Geometry: final body of the model. Coordinates: model frame, mm. A direction names the side the tool comes from. Round coordinates to 2 decimals unless told otherwise and drop trailing zeros. Loops run counter-clockwise (first coordinate to the right, second up) from the corner with the lowest first, then second, coordinate; pieces in that order, holes last. Notation, with made-up numbers: (67.25, 4) - (126.25, 4) arc R24 ccw to (126.25, 40) - close; hole circle Ø5 at (-21.75, 76.5). An arc over 180 degrees is marked (long way). Answer as CSV lines item,"result".
from build123d import *

# Parameters (mm, degrees)
SKETCH1_W           = 76.2
SKETCH1_H           = 50.8
BOSS_EXTRUDE2_DEPTH = 1016
SKETCH2_R           = 25.4
CUT_EXTRUDE1_DEPTH  = 1016
FILLET1_R           = 25.4
SKETCH3_R           = 12.7
CUT_EXTRUDE2_DEPTH  = 254
SKETCH4_W           = 38.1
SKETCH4_H           = 50.8
CUT_EXTRUDE3_DEPTH  = 254
SKETCH5_W           = 38.1
SKETCH5_H           = 25.4
CUT_EXTRUDE4_DEPTH  = 254
FILLET2_R           = 25.4


with BuildPart() as part:
    # Sketch1 → Boss-Extrude2 (new body)
    with BuildSketch(Plane(origin=(0, 0, 0), x_dir=(1, 0, 0), z_dir=(0, 1, 0))):
        with Locations((38.1, -25.4)):
            Rectangle(SKETCH1_W, SKETCH1_H)
    extrude(amount=BOSS_EXTRUDE2_DEPTH)

    # Sketch2 → Cut-Extrude1 (cut)
    with BuildSketch(Plane.XY.offset(50.8)):
        with Locations((38.1, 965.2)):
            Circle(SKETCH2_R)
    extrude(amount=-CUT_EXTRUDE1_DEPTH, mode=Mode.SUBTRACT)

    # Fillet1
    fillet1_edges = [part.edges().sort_by_distance(p)[0] for p in [
        (76.2, 1016, 25.4),
        (0, 1016, 25.4),
    ]]
    fillet(fillet1_edges, radius=FILLET1_R)

    # Sketch3 → Cut-Extrude2 (cut)
    with BuildSketch(Plane.XY.offset(50.8)):
        with Locations((38.1, 25.4)):
            Circle(SKETCH3_R)
    extrude(amount=-CUT_EXTRUDE2_DEPTH, mode=Mode.SUBTRACT)

    # Sketch4 → Cut-Extrude3 (cut)
    with BuildSketch(Plane.ZY):
        with Locations((25.4, 25.4)):
            Rectangle(SKETCH4_W, SKETCH4_H)
    extrude(amount=-CUT_EXTRUDE3_DEPTH, mode=Mode.SUBTRACT)

    # Sketch5 → Cut-Extrude4 (cut)
    with BuildSketch(Plane.ZY):
        with Locations((25.4, 63.5)):
            Rectangle(SKETCH5_W, SKETCH5_H)
    extrude(amount=-CUT_EXTRUDE4_DEPTH, mode=Mode.SUBTRACT)

    # Fillet2
    fillet2_edges = [part.edges().sort_by_distance(p)[0] for p in [
        (0, 0, 47.625),
        (76.2, 0, 3.175),
        (76.2, 0, 47.625),
        (0, 0, 3.175),
    ]]
    fillet(fillet2_edges, radius=FILLET2_R)


solid = part.part
(1) Section C-C (x = 38.1). Output: boundary loops of the cut face in (y, z).
Findings below:
outline,"(0, 0) - (12.7, 0) - (12.7, 6.35) - (0, 6.35) - close; (0, 44.45) - (12.7, 44.45) - (12.7, 50.8) - (0, 50.8) - close; (38.1, 0) - (939.8, 0) - (939.8, 50.8) - (38.1, 50.8) - (38.1, 44.45) - (76.2, 44.45) - (76.2, 6.35) - (38.1, 6.35) - close; (990.6, 0) - (1016, 0) - (1016, 50.8) - (990.6, 50.8) - close"
(2) Access query for faces 1 (the face through (76.2, 501, 26)), 2 (the face through (38, 46, 6.35)). Directions: +Z, -Z, +X, -X, +Y, -Y. A direction counts if a zero-diameter tool reaches every point of the face in a straight line with its end or side. Return the directions, or none.
Findings below:
face 1,"+Z, -Z, +X, +Y, -Y"
face 2,"+X, -X, -Y"
(3) Section B-B (z = 22). Output: boundary loops of the cut face in (x, y), and give its area (3 significant figures).
Findings below:
outline,"(0, 76.2) - (76.2, 76.2) - (76.2, 990.6) arc R25.4 ccw to (50.8, 1016) - (25.4, 1016) arc R25.4 ccw to (0, 990.6) - close; hole circle Ø50.8 at (38.1, 965.2)"
area,"69,300 mm2"
(4) Pin query (flat end, axial travel): P1, Ø12, axis at x = 61, z = 6, coming from the -Y side; P2, Ø2, axis at x = 19, z = 7, coming from the -Y side; P3, Ø10, axis at x = 64, z = 29, coming from the -Y side. Return the tip coordinate at first contact, or that it passes through.
Findings below:
P1,"y = 0.35"
P2,"y = 0.63"
P3,"y = 76.2"
(5) Draft query along Z for faces 3 (the face through (38, 76.2, 25)), 4 (the face through (44.927, 36.109, 3.219)), 5 (the face through (38, 501, 50.8)). Return one class per face: pulls with the +Z half, pulls with the -Z half, needs draft (parallel to the pull), parting line crosses it, or undercut.
Findings below:
face 3,"undercut"
face 4,"needs draft"
face 5,"pulls with the +Z half"
(6) Material intervals for line 1 along Y through (x, z) = (38.1, 48); line 2 along X through (y, z) = (25, 2); line 3 along Y through (x, z) = (38.1, 22), sorted ascending.
Findings below:
line 1,"0 to 12.7, 38.1 to 939.8, 990.6 to 1016"
line 2,"0 to 25.41, 50.79 to 76.2"
line 3,"76.2 to 939.8, 990.6 to 1016"
(7) Section A-A (y = 965.2). Output: boundary loops of the cut face in (x, z).
Findings below:
outline,"(0, 0) - (12.7, 0) - (12.7, 50.8) - (0, 50.8) - close; (63.5, 0) - (76.2, 0) - (76.2, 50.8) - (63.5, 50.8) - close"
